Geometry check sheet. Reference: the model listing, model coordinates, mm. Give positions to 0.01 mm unless a question says otherwise; leave off trailing zeros. Write each loop counter-clockwise with the first axis right and the second up, starting at its lowest first coordinate (ties: lowest second). Pieces come first, ordered by that corner, then holes. Notation, with made-up numbers: (-16.5, -29.75) -> (20.5, -29.75) arc R35 cw to (20.5, 4.25) -> close; hole circle Ø6 at (12.25, 23.5). An arc over 180 degrees is marked (long way). One line per item, written item: value.
from build123d import *

# Parameters (mm, degrees)
F0_W     = 404
F0_H     = 145
F2_DEPTH = 3
F1_R     = 2.5
F1_R_2   = 11
F1_R_3   = 1.8
F1_R_4   = 1.75
F1_W     = 53.3
F1_H     = 13
F1_W_2   = 7
F1_H_2   = 14.5
F1_R_5   = 1.5
F3_DEPTH = 25


with BuildPart() as f2:
    # F0 (on Top) → F2 (new body)
    with BuildSketch(Plane.XY):
        with Locations((-14.1859020234, -7.6260944492)):
            Rectangle(F0_W, F0_H)
    extrude(amount=-F2_DEPTH)

    # F1 (on Top) → F3 (cut)
    with BuildSketch(Plane.XY):
        with Locations((-210.1859020234, -68.1260944492)):
            Circle(F1_R)
        with BuildLine():
            Line((-135.1859020234, 49.1823275357), (-135.1859020234, 40.5654835659))
            ThreePointArc((-135.1859020234, 40.5654835659), (-128.3859020234, 36.8239055508), (-121.5859020234, 40.5654835659))
            Line((-121.5859020234, 40.5654835659), (-121.5859020234, 49.1823275357))
            ThreePointArc((-121.5859020234, 49.1823275357), (-128.3859020234, 52.9239055508), (-135.1859020234, 49.1823275357))
        make_face()
        with BuildLine():
            ThreePointArc((-22.25, -52.9147846764), (-11.3343496313, -46.8414689631), (-7, -35.1260944492))
            ThreePointArc((-7, -35.1260944492), (-36.7153745139, -21.4604440805), (-27.75, -52.9147846764))
            Line((-27.75, -52.9147846764), (-27.75, -31.4030106551))
            Line((-27.75, -31.4030106551), (-22.25, -31.4030106551))
            Line((-22.25, -31.4030106551), (-22.25, -52.9147846764))
        make_face()
        with BuildLine():
            Line((-27.75, -31.4030106551), (-27.75, -52.9147846764))
            ThreePointArc((-27.75, -52.9147846764), (-25, -53.1260944492), (-22.25, -52.9147846764))
            Line((-22.25, -52.9147846764), (-22.25, -31.4030106551))
            Line((-22.25, -31.4030106551), (-27.75, -31.4030106551))
        make_face()
        with BuildLine():
            ThreePointArc((-22.25, -52.9147846764), (-25, -53.1260944492), (-27.75, -52.9147846764))
            Line((-27.75, -52.9147846764), (-27.75, -56.6260944492))
            Line((-27.75, -56.6260944492), (-22.25, -56.6260944492))
            Line((-22.25, -56.6260944492), (-22.25, -52.9147846764))
        make_face()
        with Locations((-25, 44.8739055508)):
            Circle(F1_R_2)
        with Locations((-40.5, 44.8739055508)):
            Circle(F1_R_3)
        with Locations((-9.5, 44.8739055508)):
            Circle(F1_R_3)
        with Locations((-210.1859020234, -48.1260944492)):
            Circle(F1_R)
        with BuildLine():
            Line((152.8140979766, 39.8739055508), (172.8140979766, 39.8739055508))
            ThreePointArc((172.8140979766, 39.8739055508), (175.6425251014, 41.045478426), (176.8140979766, 43.8739055508))
            Line((176.8140979766, 43.8739055508), (176.8140979766, 55.8739055508))
            ThreePointArc((176.8140979766, 55.8739055508), (175.6425251014, 58.7023326755), (172.8140979766, 59.8739055508))
            Line((172.8140979766, 59.8739055508), (152.8140979766, 59.8739055508))
            ThreePointArc((152.8140979766, 59.8739055508), (149.9856708519, 58.7023326755), (148.8140979766, 55.8739055508))
            Line((148.8140979766, 55.8739055508), (148.8140979766, 43.8739055508))
            ThreePointArc((148.8140979766, 43.8739055508), (149.9856708519, 41.045478426), (152.8140979766, 39.8739055508))
        make_face()
        with Locations((142.8140979766, 49.8739055508)):
            Circle(F1_R_4)
        with Locations((182.8140979766, 49.8739055508)):
            Circle(F1_R_4)
        with Locations((-174.0359020234, -51.6260944492)):
            Rectangle(F1_W, F1_H)
        with Locations((-114.3359020234, -51.6260944492)):
            Rectangle(F1_W, F1_H)
        with Locations((-200.6859020234, 44.8239055508)):
            Rectangle(F1_W_2, F1_H_2)
        with Locations((-200.6859020234, 59.8739055508)):
            Circle(F1_R_5)
        with Locations((-200.6859020234, 29.7739055508)):
            Circle(F1_R_5)
        with Locations((-173.6859020234, 44.8239055508)):
            Rectangle(F1_W_2, F1_H_2)
        with Locations((-173.6859020234, 59.8739055508)):
            Circle(F1_R_5)
        with Locations((-173.6859020234, 29.7739055508)):
            Circle(F1_R_5)
        with BuildLine():
            Line((-91.5859020234, 49.1823275357), (-91.5859020234, 40.5654835659))
            ThreePointArc((-91.5859020234, 40.5654835659), (-84.7859020234, 36.8239055508), (-77.9859020234, 40.5654835659))
            Line((-77.9859020234, 40.5654835659), (-77.9859020234, 49.1823275357))
            ThreePointArc((-77.9859020234, 49.1823275357), (-84.7859020234, 52.9239055508), (-91.5859020234, 49.1823275357))
        make_face()
    extrude(amount=-F3_DEPTH, mode=Mode.SUBTRACT)


solid = f2.part
1) Sectioned sample at C-C on z = -0.6. Give the number of separate pieces and of enclosed holes in the cut face, plus the area to 3 significant figures.
Verdict:
separate pieces: 1
enclosed holes: 19
area: 54,500 mm^2
2) Scan lines: probe 1 along Y at (x, z) = (-30.5, -2); probe 2 along X at (y, z) = (-35.5, -2.8); probe 3 along Y at (x, z) = (-21, -0.15). Record each from-to range of solid material in increasing order.
Verdict:
probe 1: -80.13 to -52.27, -17.99 to 35.35, 54.4 to 64.87
probe 2: -216.19 to -43, -7 to 187.81
probe 3: -80.13 to -52.68, -17.58 to 34.63, 55.12 to 64.87
3) Mould release check, pull along Y, two halves, no side actions. Record for faces 1 (the flat face through (-17, -7, 0)), 2 (the cylindrical face through (-14.51, 48.18, -1.48)): released by +Y, released by -Y, zero draft, split by the parting line, or undercut.
Verdict:
face 1: zero draft
face 2: undercut
4) Sectioned sample at A-A on x = 160. Record the cut outline in (y, z), plus the area to 3 significant figures.
Verdict:
outline: (-80.13, -3) -> (39.87, -3) -> (39.87, 0) -> (-80.13, 0) -> close; (59.87, -3) -> (64.87, -3) -> (64.87, 0) -> (59.87, 0) -> close
area: 375 mm^2
5) Sectioned sample at B-B on y = -24. Record the cut outline in (x, z), plus the area to 3 significant figures.
Verdict:
outline: (-216.19, -3) -> (-39.15, -3) -> (-39.15, 0) -> (-216.19, 0) -> close; (-10.85, -3) -> (187.81, -3) -> (187.81, 0) -> (-10.85, 0) -> close
area: 1,130 mm^2
